from build123d import *

# Parameters (mm, degrees)
F1_DEPTH = 9.525
F2_R     = 2.667
F4_DEPTH = 25.401
F5_W     = 11.42873
F5_H     = 9.652
F6_DEPTH = 15.876


with BuildPart() as f1:
    # F0 (on Top) → F1 (new body, symmetric)
    with BuildSketch(Plane.XY):
        with BuildLine():
            ThreePointArc((-12.824485, 0.254), (0, 12.827), (12.824485, 0.254))
            Line((12.824485, 0.254), (25.39873, 0.254))
            ThreePointArc((25.39873, 0.254), (0, 25.4), (-25.39873, 0.254))
            Line((-25.39873, 0.254), (-12.824485, 0.254))
        make_face()
    extrude(amount=F1_DEPTH, both=True)

    # F2 (on Front) → F4 (cut, through all)
    with BuildSketch(Plane.XZ):
        with Locations((-19.05, 0)):
            Circle(F2_R)
        with Locations((19.05, 0)):
            Circle(F2_R)
    extrude(amount=-F4_DEPTH, mode=Mode.SUBTRACT)

    # F5 (on offset) → F6 (cut, through all)
    with BuildSketch(Plane.XZ.offset(-9.525)):
        with Locations((19.684365, 0)):
            Rectangle(F5_W, F5_H)
        with Locations((-19.684365, 0)):
            Rectangle(F5_W, F5_H)
    extrude(amount=-F6_DEPTH, mode=Mode.SUBTRACT)


solid = f1.part
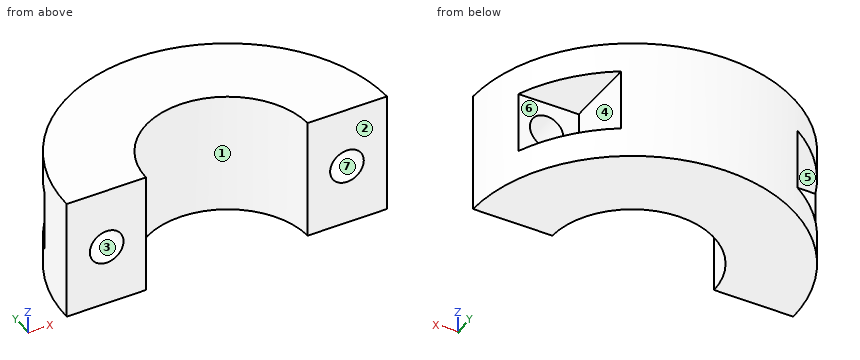
Verification items for the finished model (mm, model axes). Face numbers are marked on the shaded views. A direction names the side the tool comes from. Coordinates: 2 decimals unless noted, no trailing zeros. Order: outer loops, then holes, each group sorted by start corner. A loop starts at its lowest first (then second) coordinate and runs counter-clockwise, first axis right, second up. Notation, with made-up numbers: M -28,33.25 L 2,33.25 A20 cw 2,37.25 Z; hole C 40,80 d8. An arc over 180 degrees is marked long. Write each question's results on one line, items separated by ' | '.
1) Section check D-D on x = 0. Record the cut outline in (y, z) (3 decimals), plus the area to 3 significant figures.
Solved:
outline: M 12.827,-9.525 L 25.4,-9.525 L 25.4,9.525 L 12.827,9.525 Z | area: 240 mm²
2) Section check A-A on z = 0. Record the cut outline in (x, y) (3 decimals).
Solved:
outline: M -25.399,0.254 L -21.717,0.254 L -21.717,9.525 L -23.546,9.525 A25.4 ccw Z; M -16.383,0.254 L -12.824,0.254 A12.827 cw 12.824,0.254 L 16.383,0.254 L 16.383,9.525 L 13.97,9.525 L 13.97,21.213 A25.4 ccw -13.97,21.213 L -13.97,9.525 L -16.383,9.525 Z; M 21.717,0.254 L 25.399,0.254 A25.4 ccw 23.546,9.525 L 21.717,9.525 Z
3) Gauge pin test, flat ends, axial feed: pin 1 Ø4 at (y, z) = (3, 0) entering from +X; pin 2 Ø10.5 at (x, z) = (-17, 1) entering from +Y; pin 3 Ø1.5 at (y, z) = (8, -1) entering from +X. Record the tip position at first contact, or that the pin passes through.
Solved:
pin 1: stops at x = 25.38 | pin 2: stops at y = 22.52 | pin 3: stops at x = 24.34
4) Section check B-B on y = 4.5. Record the cut outline in (x, z) (3 decimals), plus the area to 3 significant figures.
Solved:
outline: M -24.998,-9.525 L -12.012,-9.525 L -12.012,9.525 L -24.998,9.525 Z; M 12.012,-9.525 L 24.998,-9.525 L 24.998,9.525 L 12.012,9.525 Z; hole C -19.05,0 d5.334; hole C 19.05,0 d5.334 | area: 450 mm²
5) Section check C-C on x = -19.05. Record the cut outline in (y, z) (3 decimals), plus the area to 3 significant figures.
Solved:
outline: M 0.254,-9.525 L 16.801,-9.525 L 16.801,-4.826 L 9.525,-4.826 L 9.525,-2.667 L 0.254,-2.667 Z; M 0.254,2.667 L 9.525,2.667 L 9.525,4.826 L 16.801,4.826 L 16.801,9.525 L 0.254,9.525 Z | area: 196 mm²
6) Release check for a two-part mould opening along X. For the marked faces 1, 2, 3 and 4 record: pulls with the +X half, pulls with the -X half, needs draft (parallel to the pull), parting line crosses it, or undercut.
Solved:
face 1: undercut | face 2: needs draft | face 3: undercut | face 4: pulls with the +X half
7) Scan lines: line 1 along X through (y, z) = (8, -1.75); line 2 along Z through (x, y) = (23, 10.25) (3 decimals); line 3 along Z through (x, y) = (-19.05, 3.5) (3 decimals). Record each from-to range of solid material in increasing order. Write a range as [from, to].
Solved:
line 1: x = [-24.11, -21.06], [-17.04, -10.03], [10.03, 17.04], [21.06, 24.11] | line 2: z = [-9.525, -4.826], [4.826, 9.525] | line 3: z = [-9.525, -2.667], [2.667, 9.525]
8) Access from +Z, -Z, +X, -X, +Y, -Y to the whole of each face (thin tool, end or side, straight path). Record for the marked faces 5, 6 and 7.
Solved:
face 5: -X, +Y | face 6: +X, +Y | face 7: +Y, -Y
